Geometry check sheet. Reference: the model listing, model coordinates, mm. A direction names the side the tool comes from. Round coordinates to 2 decimals unless told otherwise and drop trailing zeros. Order: outer loops, then holes, each group sorted by start corner. A loop starts at its lowest first (then second) coordinate and runs counter-clockwise, first axis right, second up. Notation, with made-up numbers: (37.25, 64.5) -> (85.25, 64.5) arc R14 cw to (85.25, 88.5) -> close; hole circle Ø4 at (51, 31.25). An arc over 180 degrees is marked (long way). Use a Markdown table: item, result. Add a question column.
Item 1: Material ranges on probe 1 along X at (y, z) = (-409, 21); probe 2 along Z at (x, y) = (29, -15); probe 3 along Z at (x, y) = (-3.5, -347.5), recorded low to high. Write a range as [from, to].
Item 2: Mould release check, pull along Z, two halves, no side actions. Record for faces 3 (the flat face through (25.4, -1058, -1)), 4 (the flat face through (31.75, -1058, -2)), 5 (the flat face through (6, -1058, -39.509)): pulls with the +Z half, pulls with the -Z half, needs draft (parallel to the pull), parting line crosses it, or undercut.
Item 3: Sectioned sample at C-C, the plane y = -857. Record the cut outline in (x, z).
Item 4: Set-up check for faces 1 (the flat face through (-12.7, -1058, -2)), 2 (the flat face through (7, -1058, 36.691)): record each of +Z, -Z, +X, -X, +Y, -Y from which the full face is reachable in a straight line by a thin tool's end or side.
Item 5: Sectioned sample at B-B, the plane x = 10. Record the cut outline in (y, z).
Item 6: Sectioned sample at A-A, the plane z = -8. Record the cut outline in (x, y), and give its area (3 significant figures).
from build123d import *

# Parameters (mm, degrees)
F1_DEPTH = 2146.4397
F2_R     = 5
F3_DEPTH = 50.801


with BuildPart() as f1:
    # F0 (on Front) → F1 (new body)
    with BuildSketch(Plane.XZ):
        with BuildLine():
            Line((25.400001, 36.691132), (-12.699999, 36.691132))
            ThreePointArc((-12.699999, 36.691132), (-17.190127, 34.83126), (-19.049999, 30.341132))
            Line((-19.049999, 30.341132), (-19.049999, -33.158868))
            ThreePointArc((-19.049999, -33.158868), (-17.190127, -37.648996), (-12.699999, -39.508868))
            Line((-12.699999, -39.508868), (25.400001, -39.508868))
            ThreePointArc((25.400001, -39.508868), (29.890129, -37.648996), (31.750001, -33.158868))
            Line((31.750001, -33.158868), (31.750001, 30.341132))
            ThreePointArc((31.750001, 30.341132), (29.890129, 34.83126), (25.400001, 36.691132))
        make_face()
        with BuildLine():
            ThreePointArc((-12.699999, 23.991132), (-10.840127, 28.48126), (-6.349999, 30.341132))
            Line((-6.349999, 30.341132), (19.050001, 30.341132))
            ThreePointArc((19.050001, 30.341132), (23.540129, 28.48126), (25.400001, 23.991132))
            Line((25.400001, 23.991132), (25.400001, -26.808868))
            ThreePointArc((25.400001, -26.808868), (23.540129, -31.298996), (19.050001, -33.158868))
            Line((19.050001, -33.158868), (-6.349999, -33.158868))
            ThreePointArc((-6.349999, -33.158868), (-10.840127, -31.298996), (-12.699999, -26.808868))
            Line((-12.699999, -26.808868), (-12.699999, 23.991132))
        make_face(mode=Mode.SUBTRACT)
    extrude(amount=F1_DEPTH)

    # F2 (on face) → F3 (cut, through all)
    with BuildSketch(Plane.YZ.offset(31.750001)):
        with Locations((-2131.4397, 21.691132)):
            Circle(F2_R)
        with Locations((-2110.6397, 21.691132)):
            Circle(F2_R)
        with Locations((-2131.4397, -24.508868)):
            Circle(F2_R)
        with Locations((-2110.6397, -24.508868)):
            Circle(F2_R)
        with Locations((-35.8, 21.691132)):
            Circle(F2_R)
        with Locations((-35.8, -24.508868)):
            Circle(F2_R)
        with Locations((-15, 21.691132)):
            Circle(F2_R)
        with Locations((-15, -24.508868)):
            Circle(F2_R)
    extrude(amount=-F3_DEPTH, mode=Mode.SUBTRACT)


solid = f1.part
Found:
| question | item | result |
|---|---|---|
| 1 | probe 1 | x = [-19.05, -12.7], [25.4, 31.75] |
| 1 | probe 2 | z = [-38.39, -29.51], [-19.51, 16.69], [26.69, 35.57] |
| 1 | probe 3 | z = [-39.51, -33.16], [30.34, 36.69] |
| 2 | face 3 | undercut |
| 2 | face 4 | needs draft |
| 2 | face 5 | pulls with the -Z half |
| 3 | outline | (-19.05, -33.16) arc R6.35 ccw to (-12.7, -39.51) -> (25.4, -39.51) arc R6.35 ccw to (31.75, -33.16) -> (31.75, 30.34) arc R6.35 ccw to (25.4, 36.69) -> (-12.7, 36.69) arc R6.35 ccw to (-19.05, 30.34) -> close; hole (-12.7, -26.81) arc R6.35 ccw to (-6.35, -33.16) -> (19.05, -33.16) arc R6.35 ccw to (25.4, -26.81) -> (25.4, 23.99) arc R6.35 ccw to (19.05, 30.34) -> (-6.35, 30.34) arc R6.35 ccw to (-12.7, 23.99) -> close |
| 4 | face 1 | +Y, -Y |
| 4 | face 2 | +Z, +X, -X, +Y, -Y |
| 5 | outline | (-2146.44, -39.51) -> (0, -39.51) -> (0, -33.16) -> (-2146.44, -33.16) -> close; (-2146.44, 30.34) -> (0, 30.34) -> (0, 36.69) -> (-2146.44, 36.69) -> close |
| 6 | outline | (-19.05, -2146.44) -> (-12.7, -2146.44) -> (-12.7, 0) -> (-19.05, 0) -> close; (25.4, -2146.44) -> (31.75, -2146.44) -> (31.75, 0) -> (25.4, 0) -> close |
| 6 | area | 27,300 mm2 |
